Work out the finished part from the listing and answer in its coordinate system (mm). Face numbers are marked on the shaded views. A direction names the side the tool comes from. Round coordinates to 2 decimals unless told otherwise and drop trailing zeros. Order: outer loops, then holes, each group sorted by start corner. A loop starts at its lowest first (then second) coordinate and runs counter-clockwise, first axis right, second up. Notation, with made-up numbers: M -26.75,18.25 L -18.75,18.25 A20 ccw -18.75,50.25 Z; hole C 47,-8 d10. An arc over 180 degrees is marked long. Return JSON: item names as keys, results as strings.
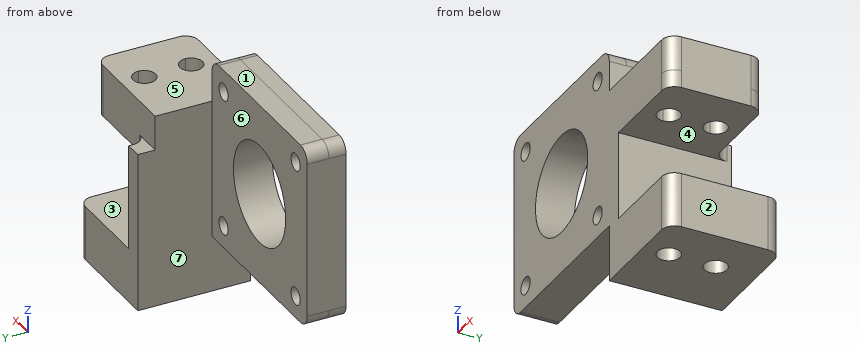
from build123d import *

# Parameters (mm, degrees)
SKETCH1_W            = 22
SKETCH1_H            = 22
BOSS_EXTRUDE2_DEPTH  = 4
SKETCH3_W            = 4
SKETCH3_H            = 22
BOSS_EXTRUDE3_DEPTH  = 24
SKETCH4_W            = 4
SKETCH4_H            = 24
BOSS_EXTRUDE4_DEPTH  = 4
SKETCH5_W            = 24
SKETCH5_H            = 4
BOSS_EXTRUDE5_DEPTH  = 24
SKETCH6_W            = 42
SKETCH6_H            = 3.943894778
BOSS_EXTRUDE6_DEPTH  = 42
SKETCH8_W            = 42
SKETCH8_H            = 42
BOSS_EXTRUDE7_DEPTH  = 4
SKETCH9_R            = 11.5
CUT_EXTRUDE1_DEPTH   = 4
SKETCH10_R           = 2.6
CUT_EXTRUDE2_DEPTH   = 4
SKETCH11_R           = 2.6
CUT_EXTRUDE3_DEPTH   = 4
FILLET1_R            = 3
SKETCH12_W           = 11.614383954
SKETCH12_H           = 9.896110461
BOSS_EXTRUDE8_DEPTH  = 4
SKETCH13_R           = 2.6
CUT_EXTRUDE5_DEPTH   = 4
SKETCH15_R           = 2
CUT_EXTRUDE7_DEPTH   = 27
SKETCH16_W           = 42
SKETCH16_H           = 42
CUT_EXTRUDE8_DEPTH   = 10
SKETCH17_W           = 42
SKETCH17_H           = 42.03828493
BOSS_EXTRUDE9_DEPTH  = 5
FILLET2_R            = 3
FILLET3_R            = 3
SKETCH18_R           = 2
SKETCH18_R_2         = 11.5
CUT_EXTRUDE9_DEPTH   = 5
SKETCH19_W           = 26
SKETCH19_H           = 22
BOSS_EXTRUDE11_DEPTH = 8
FILLET4_R            = 3
FILLET5_R            = 3
SKETCH20_W           = 4
SKETCH20_H           = 20
BOSS_EXTRUDE12_DEPTH = 26
SKETCH21_W           = 4
SKETCH21_H           = 26
BOSS_EXTRUDE13_DEPTH = 13
SKETCH25_W           = 12.6
SKETCH25_H           = 26
BOSS_EXTRUDE15_DEPTH = 22
FILLET8_R            = 3
FILLET9_R            = 3
SKETCH27_R           = 2.6
CUT_EXTRUDE10_DEPTH  = 22
SKETCH28_R           = 2.6
CUT_EXTRUDE11_DEPTH  = 46.0000001


with BuildPart() as part:
    # Sketch1 → Boss-Extrude2 (new body)
    with BuildSketch(Plane.XY):
        Rectangle(SKETCH1_W, SKETCH1_H)
    extrude(amount=BOSS_EXTRUDE2_DEPTH)

    # Sketch3 → Boss-Extrude3 (add)
    with BuildSketch(Plane.XY.offset(4)):
        with Locations((-13, 0)):
            Rectangle(SKETCH3_W, SKETCH3_H)
    extrude(amount=-BOSS_EXTRUDE3_DEPTH)

    # Sketch4 → Boss-Extrude4 (add)
    with BuildSketch(Plane(origin=(0, 11, 0), x_dir=(1, 0, 0), z_dir=(0, 1, 0))):
        with Locations((-13, 8)):
            Rectangle(SKETCH4_W, SKETCH4_H)
    extrude(amount=BOSS_EXTRUDE4_DEPTH)

    # Sketch5 → Boss-Extrude5 (add)
    with BuildSketch(Plane(origin=(-11, 0, 0), x_dir=(0, 0, -1), z_dir=(1, 0, 0))):
        with Locations((8, 13)):
            Rectangle(SKETCH5_W, SKETCH5_H)
    extrude(amount=-BOSS_EXTRUDE5_DEPTH)

    # Sketch6 → Boss-Extrude6 (add)
    with BuildSketch(Plane.ZY.offset(15)):
        with Locations((1, -9.028052611)):
            Rectangle(SKETCH6_W, SKETCH6_H)
    extrude(amount=BOSS_EXTRUDE6_DEPTH)

    # Sketch8 → Boss-Extrude7 (add)
    with BuildSketch(Plane(origin=(0, 15, 0), x_dir=(1, 0, 0), z_dir=(0, 1, 0))):
        with Locations((-36, -1)):
            Rectangle(SKETCH8_W, SKETCH8_H)
    extrude(amount=-BOSS_EXTRUDE7_DEPTH)

    # Sketch9 → Cut-Extrude1 (cut)
    with BuildSketch(Plane.XZ.offset(11)):
        with Locations((-36, 1)):
            Circle(SKETCH9_R)
    extrude(amount=-CUT_EXTRUDE1_DEPTH, mode=Mode.SUBTRACT)

    # Sketch10 → Cut-Extrude2 (cut)
    with BuildSketch(Plane(origin=(0, 15, 0), x_dir=(1, 0, 0), z_dir=(0, 1, 0))):
        with Locations((-34, -1)):
            Circle(SKETCH10_R)
    extrude(amount=-CUT_EXTRUDE2_DEPTH, mode=Mode.SUBTRACT)

    # Sketch11 → Cut-Extrude3 (cut)
    with BuildSketch(Plane.XY.offset(4)):
        with Locations((0, 5.660439733)):
            Circle(SKETCH11_R)
        with Locations((0, -5.136008772)):
            Circle(SKETCH11_R)
    extrude(amount=-CUT_EXTRUDE3_DEPTH, mode=Mode.SUBTRACT)

    # Fillet1
    fillet1_edges = [part.edges().sort_by_distance(p)[0] for p in [
        (-11, 2, -20),
        (-11, 11, 2),
        (-15, -9.028052611, 22),
        (-57, -9.028052611, -20),
        (-57, -9.028052611, 22),
        (11, -11, 2),
        (11, 11, 2),
        (-57, 13, 22),
        (-57, 13, -20),
        (-15, 13, 22),
    ]]
    fillet(fillet1_edges, radius=FILLET1_R)

    # Sketch12 → Boss-Extrude8 (add)
    with BuildSketch(Plane(origin=(0, 15, 0), x_dir=(1, 0, 0), z_dir=(0, 1, 0))):
        with Locations((-34.256477643, -1.105652727)):
            Rectangle(SKETCH12_W, SKETCH12_H)
    extrude(amount=-BOSS_EXTRUDE8_DEPTH)

    # Sketch13 → Cut-Extrude5 (cut)
    with BuildSketch(Plane.XZ.offset(-11)):
        with Locations((-36, 1)):
            Circle(SKETCH13_R)
    extrude(amount=-CUT_EXTRUDE5_DEPTH, mode=Mode.SUBTRACT)

    # Sketch15 → Cut-Extrude7 (cut, through all)
    with BuildSketch(Plane.XZ.offset(11)):
        with Locations((-20.125452762, 16.874547238)):
            Circle(SKETCH15_R)
        with Locations((-51.874547238, 16.874547238)):
            Circle(SKETCH15_R)
        with Locations((-51.874547238, -14.874547238)):
            Circle(SKETCH15_R)
        with Locations((-20.125452762, -14.874547238)):
            Circle(SKETCH15_R)
    extrude(amount=-CUT_EXTRUDE7_DEPTH, mode=Mode.SUBTRACT)

    # Sketch16 → Cut-Extrude8 (cut)
    with BuildSketch(Plane.XZ.offset(-11)):
        with Locations((-36, 1)):
            Rectangle(SKETCH16_W, SKETCH16_H)
    extrude(amount=-CUT_EXTRUDE8_DEPTH, mode=Mode.SUBTRACT)

    # Sketch17 → Boss-Extrude9 (add)
    with BuildSketch(Plane(origin=(0, -7.056105222, 0), x_dir=(1, 0, 0), z_dir=(0, 1, 0))):
        with Locations((-36, -1.019142465)):
            Rectangle(SKETCH17_W, SKETCH17_H)
    extrude(amount=BOSS_EXTRUDE9_DEPTH)

    # Fillet2
    fillet2_edges = [part.edges().sort_by_distance(p)[0] for p in [
        (-15, -4.556105222, 22.03828493),
    ]]
    fillet(fillet2_edges, radius=FILLET2_R)

    # Fillet3
    fillet3_edges = [part.edges().sort_by_distance(p)[0] for p in [
        (-57, -4.556105222, -20),
        (-57, -4.556105222, 22.03828493),
    ]]
    fillet(fillet3_edges, radius=FILLET3_R)

    # Sketch18 → Cut-Extrude9 (cut)
    with BuildSketch(Plane.XZ.offset(7.056105222)):
        with Locations((-20.125452762, 16.874547238)):
            Circle(SKETCH18_R)
        with Locations((-51.874547238, 16.874547238)):
            Circle(SKETCH18_R)
        with Locations((-51.874547238, -14.874547238)):
            Circle(SKETCH18_R)
        with Locations((-20.125452762, -14.874547238)):
            Circle(SKETCH18_R)
        with Locations((-36, 1)):
            Circle(SKETCH18_R_2)
    extrude(amount=-CUT_EXTRUDE9_DEPTH, mode=Mode.SUBTRACT)

    # Sketch19 → Boss-Extrude11 (add)
    with BuildSketch(Plane.XY.offset(4)):
        with Locations((-2, 0)):
            Rectangle(SKETCH19_W, SKETCH19_H)
    extrude(amount=BOSS_EXTRUDE11_DEPTH)

    # Fillet4
    fillet4_edges = [part.edges().sort_by_distance(p)[0] for p in [
        (11, 11, 8),
    ]]
    fillet(fillet4_edges, radius=FILLET4_R)

    # Fillet5
    fillet5_edges = [part.edges().sort_by_distance(p)[0] for p in [
        (11, -11, 8),
    ]]
    fillet(fillet5_edges, radius=FILLET5_R)

    # Sketch20 → Boss-Extrude12 (add, through all)
    with BuildSketch(Plane(origin=(0, 15, 0), x_dir=(1, 0, 0), z_dir=(0, 1, 0))):
        with Locations((-13, 10)):
            Rectangle(SKETCH20_W, SKETCH20_H)
    extrude(amount=-BOSS_EXTRUDE12_DEPTH)

    # Sketch21 → Boss-Extrude13 (add)
    with BuildSketch(Plane(origin=(0, 0, -20), x_dir=(-1, 0, 0), z_dir=(0, 0, -1))):
        with Locations((13, 2)):
            Rectangle(SKETCH21_W, SKETCH21_H)
    extrude(amount=BOSS_EXTRUDE13_DEPTH)

    # Sketch25 → Boss-Extrude15 (add)
    with BuildSketch(Plane(origin=(-11, 0, 0), x_dir=(0, 0, -1), z_dir=(1, 0, 0))):
        with Locations((26.7, 2)):
            Rectangle(SKETCH25_W, SKETCH25_H)
    extrude(amount=BOSS_EXTRUDE15_DEPTH)

    # Fillet8
    fillet8_edges = [part.edges().sort_by_distance(p)[0] for p in [
        (11, 15, -26.7),
    ]]
    fillet(fillet8_edges, radius=FILLET8_R)

    # Fillet9
    fillet9_edges = [part.edges().sort_by_distance(p)[0] for p in [
        (11, -11, -26.7),
    ]]
    fillet(fillet9_edges, radius=FILLET9_R)

    # Sketch27 → Cut-Extrude10 (cut)
    with BuildSketch(Plane(origin=(0, 0, 0), x_dir=(-1, 0, 0), z_dir=(0, 0, -1))):
        with Locations((0, 5.660439733)):
            Circle(SKETCH27_R)
        with Locations((0, -5.136008772)):
            Circle(SKETCH27_R)
    extrude(amount=-CUT_EXTRUDE10_DEPTH, mode=Mode.SUBTRACT)

    # Sketch28 → Cut-Extrude11 (cut, through all)
    with BuildSketch(Plane.XY.offset(12)):
        with Locations((0, 5.660439733)):
            Circle(SKETCH28_R)
        with Locations((0, -5.136008772)):
            Circle(SKETCH28_R)
    extrude(amount=-CUT_EXTRUDE11_DEPTH, mode=Mode.SUBTRACT)


solid = part.part
Item 1: Find section B-B (z = 1). Determine the outline of the cut face in (x, y), plus the area to 3 significant figures.
Output:
{"outline": "M -57,-11 L -47.5,-11 L -47.5,-2.06 L -57,-2.06 Z; M -24.5,-11 L 8,-11 A3 ccw 11,-8 L 11,8 A3 ccw 8,11 L -8,11 A3 cw -11,14 L -11,15 L -15,15 L -15,-2.06 L -24.5,-2.06 Z; hole C 0,-5.14 d5.2; hole C 0,5.66 d5.2", "area": "714 mm^2"}
Item 2: Each of these flat-tipped pins is pushed along its axis until it touches: pin 1 (3 mm diameter, centred on x = -45.5, z = 13, fed in from +Y); pin 2 (8.5 mm diameter, centred on x = 0, y = 5.66, fed in from +Z); pin 3 (2 mm diameter, centred on x = -42.5, y = -8.5, fed in from +Z). Where does it stop, or does it pass through?
Output:
{"pin 1": "stops at y = -2.06", "pin 2": "stops at z = 12", "pin 3": "stops at z = 22"}
Item 3: Which of the six approach directions +Z, -Z, +X, -X, +Y, -Y give full straight-line access (tool end or side, diameter ignored) to the marked faces 4, 5, 6 and 7?
Output:
{"face 4": "+X, +Y, -Y", "face 5": "+Z, +X, +Y, -Y", "face 6": "+Z, -Z, -X, +Y", "face 7": "-Z, -X, +Y"}
Item 4: The mould has two halves that part along Z. Classify the marked faces 1, 2 and 3: pulls with the +Z half, pulls with the -Z half, needs draft (parallel to the pull), parting line crosses it, or undercut.
Output:
{"face 1": "pulls with the +Z half", "face 2": "needs draft", "face 3": "undercut"}
Item 5: Consider line 1 along Y through (x, z) = (0, -25.25); line 2 along X through (y, z) = (-5, -26); line 3 along Z through (x, y) = (-10, -5.25). Determine where each line is inside the solid, lowest interval first. Write a range as [from, to].
Output:
{"line 1": "y = [-11, -7.74], [-2.54, 3.06], [8.26, 15]", "line 2": "x = [-15, -2.6], [2.6, 11]", "line 3": "z = [-33, -20.4], [0, 12]"}
Item 6: Find section C-C (x = 0). Determine the outline of the cut face in (y, z).
Output:
{"outline": "M -11,-33 L -7.74,-33 L -7.74,-20.4 L -11,-20.4 Z; M -11,0 L -7.74,0 L -7.74,12 L -11,12 Z; M -2.54,-33 L 3.06,-33 L 3.06,-20.4 L -2.54,-20.4 Z; M -2.54,0 L 3.06,0 L 3.06,12 L -2.54,12 Z; M 8.26,-33 L 15,-33 L 15,-20.4 L 8.26,-20.4 Z; M 8.26,0 L 11,0 L 11,12 L 8.26,12 Z"}
Item 7: Find section D-D (z = -16). Determine the outline of the cut face in (x, y), plus the area to 3 significant figures.
Output:
{"outline": "M -57,-11 L -53.53,-11 L -53.53,-2.06 L -57,-2.06 Z; M -50.22,-11 L -21.78,-11 L -21.78,-2.06 L -50.22,-2.06 Z; M -18.47,-11 L -11,-11 L -11,15 L -15,15 L -15,-2.06 L -18.47,-2.06 Z", "area": "420 mm^2"}
